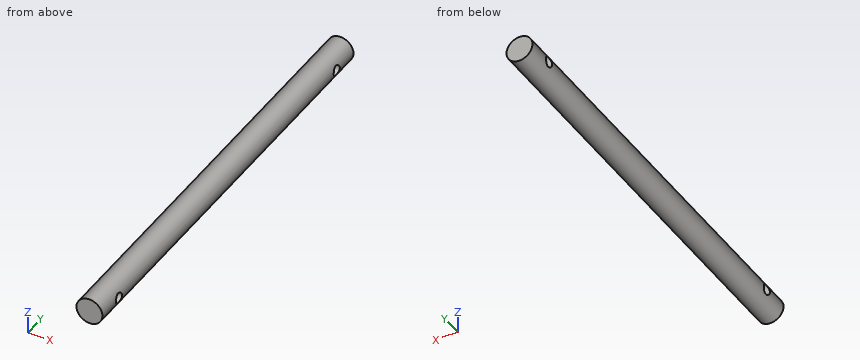
from build123d import *

# Parameters (mm, degrees)
SKETCH1_R           = 3.9624
BOSS_EXTRUDE1_DEPTH = 65.0875
SKETCH2_W           = 32.020580586
SKETCH2_H           = 1.5875


with BuildPart() as part:
    # Sketch1 → Boss-Extrude1 (new body, symmetric)
    with BuildSketch(Plane(origin=(0, 0, 0), x_dir=(1, 0, 0), z_dir=(0, 1, 0))):
        Circle(SKETCH1_R)
    extrude(amount=BOSS_EXTRUDE1_DEPTH, both=True)

    # Sketch2 → Cut-Revolve1 (revolve, cut)
    with BuildSketch(Plane.XY):
        with Locations((-1.023553281, 57.21985)):
            Rectangle(SKETCH2_W, SKETCH2_H)
    cut_revolve1 = revolve(axis=Axis((14.986737012, 56.4261, 0), (-1, 0, 0)), mode=Mode.SUBTRACT)

    # Mirror1: Cut-Revolve1 across plane
    add(cut_revolve1.mirror(Plane.ZX), mode=Mode.SUBTRACT)


solid = part.part
Model file for the job. Use its own axes, mm. Coordinates: 2 decimals unless noted, no trailing zeros. Order: outer loops, then holes, each group sorted by start corner. A loop starts at its lowest first (then second) coordinate and runs counter-clockwise, first axis right, second up. Notation, with made-up numbers: M -11.75,-31 L 6.25,-31 A14 cw 6.25,-13 Z; hole C 54.25,34.5 d10. An arc over 180 degrees is marked long. Return JSON: item names as keys, results as strings.
1. Saw through at B-B (x = 0). Give the cut face in (y, z) (1 decimal), and give its area (3 significant figures).
Ans:
{"outline": "M -65.1,-4 L 65.1,-4 L 65.1,4 L -65.1,4 Z; hole C -56.4,0 d3.2; hole C 56.4,0 d3.2", "area": "1,020 mm^2"}
2. Saw through at A-A (z = 0). Give the cut face in (x, y).
Ans:
{"outline": "M -3.96,-65.09 L 3.96,-65.09 L 3.96,-58.01 L -3.96,-58.01 Z; M -3.96,-54.84 L 3.96,-54.84 L 3.96,54.84 L -3.96,54.84 Z; M -3.96,58.01 L 3.96,58.01 L 3.96,65.09 L -3.96,65.09 Z"}
3. Saw through at C-C (y = -53). Give the cut face in (x, z).
Ans:
{"outline": "C 0,0 d7.92"}
4. Flat gauge pins, fed straight in: pin 1 (1.5 mm diameter, centred on x = 1, y = -40, fed in from +Z); pin 2 (3 mm diameter, centred on y = -56.43, z = 0, fed in from -X); pin 3 (3.5 mm diameter, centred on y = 56.43, z = 0, fed in from -X); pin 4 (1.5 mm diameter, centred on x = -1.5, y = -31, fed in from -Z). Where does each tip first touch, or does it go through?
Ans:
{"pin 1": "z = 3.95", "pin 2": "through", "pin 3": "x = -3.96", "pin 4": "z = -3.89"}
5. Drill centre lines: probe 1 along Y at (x, z) = (1.75, 0); probe 2 along Y at (x, z) = (-3.5, 1); probe 3 along X at (y, z) = (18.5, 0.25). Where is each one in solid material? Low to high.
Ans:
{"probe 1": "-65.09 to -58.01, -54.84 to 54.84, 58.01 to 65.09", "probe 2": "-65.09 to -57.66, -55.19 to 55.19, 57.66 to 65.09", "probe 3": "-3.95 to 3.95"}
